```python
from build123d import *

# Parameters (mm, degrees)
SKETCH1_W           = 267
SKETCH1_H           = 350.4
SKETCH1_R           = 2.1
SKETCH1_R_2         = 2.5
SKETCH1_R_3         = 1.59
SKETCH1_R_4         = 12.5
SKETCH1_W_2         = 33
SKETCH1_H_2         = 90
BOSS_EXTRUDE1_DEPTH = 5
SKETCH12_W          = 267
SKETCH12_H          = 5
CUT_EXTRUDE2_DEPTH  = 83
CUT_EXTRUDE3_DEPTH  = 6
SKETCH15_W          = 28.794476706
SKETCH15_H          = 22.5
SKETCH15_W_2        = 7.746360579
CUT_EXTRUDE4_DEPTH  = 10


with BuildPart() as part:
    # Sketch1 → Boss-Extrude1 (new body)
    with BuildSketch(Plane.XY):
        with Locations((133.5, -175.2)):
            Rectangle(SKETCH1_W, SKETCH1_H)
        with Locations((133.5, -45)):
            Circle(SKETCH1_R, mode=Mode.SUBTRACT)
        with Locations((133.5, -4)):
            Circle(SKETCH1_R, mode=Mode.SUBTRACT)
        with Locations((263, -119.5)):
            Circle(SKETCH1_R_2, mode=Mode.SUBTRACT)
        with Locations((263, -170.5)):
            Circle(SKETCH1_R_2, mode=Mode.SUBTRACT)
        with Locations((196.56, -129.375)):
            Circle(SKETCH1_R_3, mode=Mode.SUBTRACT)
        with Locations((196.56, -160.625)):
            Circle(SKETCH1_R_3, mode=Mode.SUBTRACT)
        with Locations((133.5, -24.5)):
            Circle(SKETCH1_R_4, mode=Mode.SUBTRACT)
        with Locations((158.46, -129.375)):
            Circle(SKETCH1_R_3, mode=Mode.SUBTRACT)
        with Locations((171.16, -129.375)):
            Circle(SKETCH1_R_3, mode=Mode.SUBTRACT)
        with Locations((183.86, -129.375)):
            Circle(SKETCH1_R_3, mode=Mode.SUBTRACT)
        with Locations((158.46, -160.625)):
            Circle(SKETCH1_R_3, mode=Mode.SUBTRACT)
        with Locations((171.16, -160.625)):
            Circle(SKETCH1_R_3, mode=Mode.SUBTRACT)
        with Locations((183.86, -160.625)):
            Circle(SKETCH1_R_3, mode=Mode.SUBTRACT)
        with Locations((83.14, -160.625)):
            Circle(SKETCH1_R_3, mode=Mode.SUBTRACT)
        with Locations((95.84, -160.625)):
            Circle(SKETCH1_R_3, mode=Mode.SUBTRACT)
        with Locations((108.54, -160.625)):
            Circle(SKETCH1_R_3, mode=Mode.SUBTRACT)
        with Locations((83.14, -129.375)):
            Circle(SKETCH1_R_3, mode=Mode.SUBTRACT)
        with Locations((95.84, -129.375)):
            Circle(SKETCH1_R_3, mode=Mode.SUBTRACT)
        with Locations((108.54, -129.375)):
            Circle(SKETCH1_R_3, mode=Mode.SUBTRACT)
        with Locations((70.44, -160.625)):
            Circle(SKETCH1_R_3, mode=Mode.SUBTRACT)
        with Locations((70.44, -129.375)):
            Circle(SKETCH1_R_3, mode=Mode.SUBTRACT)
        with Locations((4, -170.5)):
            Circle(SKETCH1_R_2, mode=Mode.SUBTRACT)
        with Locations((4, -119.5)):
            Circle(SKETCH1_R_2, mode=Mode.SUBTRACT)
        with Locations((219.06, -145)):
            Rectangle(SKETCH1_W_2, SKETCH1_H_2, mode=Mode.SUBTRACT)
        with BuildLine():
            Line((163.2225, -129.375), (163.2225, -149.054634918))
            ThreePointArc((163.2225, -149.054634918), (164.81, -149.140223925), (166.3975, -149.054634918))
            Line((166.3975, -149.054634918), (166.3975, -129.375))
            ThreePointArc((166.3975, -129.375), (164.81, -127.7875), (163.2225, -129.375))
        make_face(mode=Mode.SUBTRACT)
        with BuildLine():
            Line((175.92, -129.375), (175.92, -149.054634918))
            ThreePointArc((175.92, -149.054634918), (177.51, -149.140492925), (179.1, -149.054634918))
            Line((179.1, -149.054634918), (179.1, -129.375))
            ThreePointArc((179.1, -129.375), (177.51, -127.785), (175.92, -129.375))
        make_face(mode=Mode.SUBTRACT)
        with BuildLine():
            Line((188.62, -129.375), (188.62, -149.054634918))
            ThreePointArc((188.62, -149.054634918), (190.21, -149.140492925), (191.8, -149.054634918))
            Line((191.8, -149.054634918), (191.8, -129.375))
            ThreePointArc((191.8, -129.375), (190.21, -127.785), (188.62, -129.375))
        make_face(mode=Mode.SUBTRACT)
        with BuildLine():
            Line((163.2225, -160.625), (163.2225, -180.304634918))
            ThreePointArc((163.2225, -180.304634918), (164.81, -180.390223925), (166.3975, -180.304634918))
            Line((166.3975, -180.304634918), (166.3975, -160.625))
            ThreePointArc((166.3975, -160.625), (164.81, -159.0375), (163.2225, -160.625))
        make_face(mode=Mode.SUBTRACT)
        with BuildLine():
            Line((175.92, -160.625), (175.92, -180.304634918))
            ThreePointArc((175.92, -180.304634918), (177.51, -180.390492925), (179.1, -180.304634918))
            Line((179.1, -180.304634918), (179.1, -160.625))
            ThreePointArc((179.1, -160.625), (177.51, -159.035), (175.92, -160.625))
        make_face(mode=Mode.SUBTRACT)
        with BuildLine():
            Line((188.62, -160.625), (188.62, -180.304634918))
            ThreePointArc((188.62, -180.304634918), (190.21, -180.390492925), (191.8, -180.304634918))
            Line((191.8, -180.304634918), (191.8, -160.625))
            ThreePointArc((191.8, -160.625), (190.21, -159.035), (188.62, -160.625))
        make_face(mode=Mode.SUBTRACT)
        with BuildLine():
            Line((103.7775, -129.375), (103.7775, -149.054634918))
            ThreePointArc((103.7775, -149.054634918), (102.19, -150.642134918), (100.6025, -149.054634918))
            Line((100.6025, -149.054634918), (100.6025, -129.375))
            ThreePointArc((100.6025, -129.375), (102.19, -127.7875), (103.7775, -129.375))
        make_face(mode=Mode.SUBTRACT)
        with BuildLine():
            Line((91.08, -129.375), (91.08, -149.054634918))
            ThreePointArc((91.08, -149.054634918), (89.49, -150.644634918), (87.9, -149.054634918))
            Line((87.9, -149.054634918), (87.9, -129.375))
            ThreePointArc((87.9, -129.375), (89.49, -127.785), (91.08, -129.375))
        make_face(mode=Mode.SUBTRACT)
        with BuildLine():
            Line((78.38, -129.375), (78.38, -149.054634918))
            ThreePointArc((78.38, -149.054634918), (76.79, -150.644634918), (75.2, -149.054634918))
            Line((75.2, -149.054634918), (75.2, -129.375))
            ThreePointArc((75.2, -129.375), (76.79, -127.785), (78.38, -129.375))
        make_face(mode=Mode.SUBTRACT)
        with BuildLine():
            Line((103.7775, -160.625), (103.7775, -180.304634918))
            ThreePointArc((103.7775, -180.304634918), (102.19, -181.892134918), (100.6025, -180.304634918))
            Line((100.6025, -180.304634918), (100.6025, -160.625))
            ThreePointArc((100.6025, -160.625), (102.19, -159.0375), (103.7775, -160.625))
        make_face(mode=Mode.SUBTRACT)
        with BuildLine():
            Line((91.08, -160.625), (91.08, -180.304634918))
            ThreePointArc((91.08, -180.304634918), (89.49, -181.894634918), (87.9, -180.304634918))
            Line((87.9, -180.304634918), (87.9, -160.625))
            ThreePointArc((87.9, -160.625), (89.49, -159.035), (91.08, -160.625))
        make_face(mode=Mode.SUBTRACT)
        with BuildLine():
            Line((78.38, -160.625), (78.38, -180.304634918))
            ThreePointArc((78.38, -180.304634918), (76.79, -181.894634918), (75.2, -180.304634918))
            Line((75.2, -180.304634918), (75.2, -160.625))
            ThreePointArc((75.2, -160.625), (76.79, -159.035), (78.38, -160.625))
        make_face(mode=Mode.SUBTRACT)
        with Locations((47.94, -145)):
            Rectangle(SKETCH1_W_2, SKETCH1_H_2, mode=Mode.SUBTRACT)
    extrude(amount=BOSS_EXTRUDE1_DEPTH)

    # Sketch12 → Cut-Extrude2 (cut)
    with BuildSketch(Plane.XZ.offset(350.4)):
        with Locations((133.5, 2.5)):
            Rectangle(SKETCH12_W, SKETCH12_H)
    extrude(amount=-CUT_EXTRUDE2_DEPTH, mode=Mode.SUBTRACT)

    # Sketch13 → Cut-Extrude3 (cut, through all)
    with BuildSketch(Plane.XY.offset(5)):
        with BuildLine():
            Line((46.750392508, -85), (26.604338358, -85))
            Line((26.604338358, -85), (26.604338358, -113))
            Line((26.604338358, -113), (0, -113))
            Line((0, -113), (0, 0))
            Line((0, 0), (105.059911457, 0))
            ThreePointArc((105.059911457, 0), (98.289212828, -57.855339059), (46.750392508, -85))
        make_face()
        with BuildLine():
            Line((267, 0), (267, -113))
            Line((267, -113), (240.395661642, -113))
            Line((240.395661642, -113), (240.395661642, -85))
            Line((240.395661642, -85), (220.249607492, -85))
            ThreePointArc((220.249607492, -85), (168.710787172, -57.855339059), (161.940088543, 0))
            Line((161.940088543, 0), (267, 0))
        make_face()
        with BuildLine():
            Line((71, -227.4), (71, -350.4))
            Line((71, -350.4), (196, -350.4))
            Line((196, -350.4), (196, -227.4))
            ThreePointArc((196, -227.4), (133.5, -164.9), (71, -227.4))
        make_face()
    extrude(amount=-CUT_EXTRUDE3_DEPTH, mode=Mode.SUBTRACT)

    # Sketch15 → Cut-Extrude4 (cut)
    with BuildSketch(Plane.XY.offset(5)):
        with Locations((94.853154155, -11.25)):
            Rectangle(SKETCH15_W, SKETCH15_H)
        with Locations((161.622787782, -11.25)):
            Rectangle(SKETCH15_W_2, SKETCH15_H)
    extrude(amount=-CUT_EXTRUDE4_DEPTH, mode=Mode.SUBTRACT)


solid = part.part
```
CAD build for the part. Positions are in the model's coordinates, mm. A direction names the side the tool comes from. Round coordinates to 2 decimals unless told otherwise and drop trailing zeros. Write each loop counter-clockwise with the first axis right and the second up, starting at its lowest first coordinate (ties: lowest second). Pieces come first, ordered by that corner, then holes. Notation, with made-up numbers: (28, -19.5) - (69, -19.5) arc R30 ccw to (69, 8.5) - close; hole circle Ø11 at (83.5, 69.5). An arc over 180 degrees is marked (long way). Return JSON: item names as keys, results as strings. Group by question number.
Item 1: Band-saw the part on C-C on y = -64.5. List the corners of the cut face in (x, z), plus the area to 3 significant figures.
Item 2: Band-saw the part on A-A on y = -106.5. List the corners of the cut face in (x, z), plus the area to 3 significant figures.
Item 3: 3-axis set-ups, long thin cutter, end or side, ignore diameter. For faces 1 (the face through (91.428, -66.206, 2.535)), 2 (the face through (79.118, -196.597, 2.535)): which of +Z, -Z, +X, -X, +Y, -Y reach the whole face in a straight line?
Item 4: Flat gauge pins, fed straight in: pin 1 Ø20 at (x, y) = (133.5, -24.5) entering from +Z; pin 2 Ø2.5 at (y, z) = (-104, 2.5) entering from +X; pin 3 Ø2 at (x, z) = (194, 1) entering from +Y; pin 4 Ø2 at (y, z) = (-238, 0.5) entering from -X. Where does each tip first touch, or does it go through?
Item 5: Probe probe 1 along Y at (x, z) = (4, 3.5); probe 2 along X at (y, z) = (-123, 0.4); probe 3 along Y at (x, z) = (83.14, 4) (3 decimals). List the from-to ranges inside material, lowest first.
Item 6: Band-saw the part on B-B on z = 3.15. State how many separate pieces and enclosed holes the cut face has, plus the area to 3 significant figures.
Item 7: Mould opens along Y. For faces 3 (the face through (145.423, -20.745, 2.465)), 4 (the face through (132, -162, 5)), 5 (the face through (133.9, -164.9, 2.5)) say: +Y half, -Y half, draft (parallel to the pull), parting line (faces both ways), or undercut.
Resolved:
{
 "1": {"outline": "(93.03, 0) - (173.97, 0) - (173.97, 5) - (93.03, 5) - close", "area": "405 mm²"},
 "2": {"outline": "(26.6, 0) - (31.44, 0) - (31.44, 5) - (26.6, 5) - close; (64.44, 0) - (202.56, 0) - (202.56, 5) - (64.44, 5) - close; (235.56, 0) - (240.4, 0) - (240.4, 5) - (235.56, 5) - close", "area": "739 mm²"},
 "3": {"face 1": "+Z, -Z, -X, +Y", "face 2": "+Z, -Z, -Y"},
 "4": {"pin 1": "passes through", "pin 2": "stops at x = 240.4", "pin 3": "stops at y = -78.75", "pin 4": "stops at x = 0"},
 "5": {"probe 1": "y = -267.4 to -173, -168 to -122, -117 to -113", "probe 2": "x = 0 to 31.44, 64.44 to 202.56, 235.56 to 267", "probe 3": "y = -190.385 to -162.215, -159.035 to -130.965, -127.785 to -73.314"},
 "6": {"separate pieces": "1", "enclosed holes": "35", "area": "34,400 mm²"},
 "7": {"face 3": "undercut", "face 4": "draft", "face 5": "-Y half"}
}
